```python
from build123d import *

# Parameters (mm, degrees)
SKETCH1_R           = 5
SKETCH1_W           = 15.28
SKETCH1_H           = 2.7
BOSS_EXTRUDE1_DEPTH = 2.7


with BuildPart() as part:
    # Sketch1 → Boss-Extrude1 (new body)
    with BuildSketch(Plane.XY):
        Polygon((38.2, 27.2), (22.92, 27.2), (22.92, 24.5), (7.64, 24.5), (7.64, 27.2), (-7.64, 27.2), (-7.64, 24.5), (-22.92, 24.5), (-22.92, 27.2), (-38.2, 27.2), (-38.2, 16.32), (-35.5, 16.32), (-35.5, 5.44), (-38.2, 5.44), (-38.2, -5.44), (-35.5, -5.44), (-35.5, -16.32), (-38.2, -16.32), (-38.2, -107.3), (-22.92, -107.3), (-22.92, -110), (-7.64, -110), (-7.64, -107.3), (7.64, -107.3), (7.64, -110), (22.92, -110), (22.92, -107.3), (38.2, -107.3), (38.2, -16.32), (35.5, -16.32), (35.5, -5.44), (38.2, -5.44), (38.2, 5.44), (35.5, 5.44), (35.5, 16.32), (38.2, 16.32), align=None)
        with Locations((26.908058417, 15.599455208)):
            Circle(SKETCH1_R, mode=Mode.SUBTRACT)
        with Locations((-15.28, -25.85)):
            Rectangle(SKETCH1_W, SKETCH1_H, mode=Mode.SUBTRACT)
        with Locations((15.28, -25.85)):
            Rectangle(SKETCH1_W, SKETCH1_H, mode=Mode.SUBTRACT)
    extrude(amount=-BOSS_EXTRUDE1_DEPTH)


solid = part.part
```
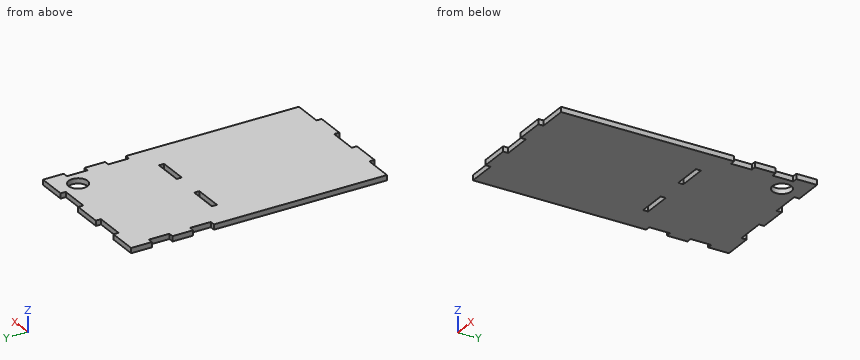
Build history of the part. All positions in model axes, mm. Round coordinates to 2 decimals unless told otherwise and drop trailing zeros. Order: outer loops, then holes, each group sorted by start corner. A loop starts at its lowest first (then second) coordinate and runs counter-clockwise, first axis right, second up. Notation, with made-up numbers: (47, 61.25) -> (57, 61.25) arc R24 cw to (57, 81.25) -> close; hole circle Ø5 at (88.25, 83). An arc over 180 degrees is marked (long way). Answer in a Markdown table with one row per item.
1) Wall check: L1, parallel to Y at x = 8, z = -1.15; L2, parallel to Y at x = 0, z = -1.9; L3, parallel to X at y = 9, z = -0.8. Give the ranges that are in metal, low to high.
Values:
| item | result |
|---|---|
| L1 | -110 to -27.2, -24.5 to 24.5 |
| L2 | -107.3 to 27.2 |
| L3 | -35.5 to 35.5 |
2) Band-saw the part on C-C on x = -5. Give the cut face in (y, z), and give its area (3 significant figures).
Values:
| item | result |
|---|---|
| outline | (-107.3, -2.7) -> (27.2, -2.7) -> (27.2, 0) -> (-107.3, 0) -> close |
| area | 363 mm2 |
3) Pin check, flat tips, straight feed: P1, Ø0.8, axis at x = 36.5, z = -1.5, coming from the -Y side; P2, Ø0.8, axis at x = 12, z = -1, coming from the +Y side. Stop position of each tip, or through.
Values:
| item | result |
|---|---|
| P1 | y = -107.3 |
| P2 | y = 24.5 |
4) Band-saw the part on A-A on x = 18. Give the cut face in (y, z), and give its area (3 significant figures).
Values:
| item | result |
|---|---|
| outline | (-110, -2.7) -> (-27.2, -2.7) -> (-27.2, 0) -> (-110, 0) -> close; (-24.5, -2.7) -> (24.5, -2.7) -> (24.5, 0) -> (-24.5, 0) -> close |
| area | 356 mm2 |
5) Band-saw the part on D-D on z = -1.7. Give the number of separate pieces and of enclosed holes in the cut face, and give its area (4 significant figures).
Values:
| item | result |
|---|---|
| separate pieces | 1 |
| enclosed holes | 3 |
| area | 10,000 mm2 |
6) Band-saw the part on B-B on y = -14.5. Give the cut face in (x, z).
Values:
| item | result |
|---|---|
| outline | (-35.5, -2.7) -> (35.5, -2.7) -> (35.5, 0) -> (-35.5, 0) -> close |
